The listing builds one solid part. Answer for the finished solid, in the listing's coordinates (mm). Face numbers are marked on the shaded views. A direction names the side the tool comes from. Coordinates: 2 decimals unless noted, no trailing zeros. Order: outer loops, then holes, each group sorted by start corner. A loop starts at its lowest first (then second) coordinate and runs counter-clockwise, first axis right, second up.
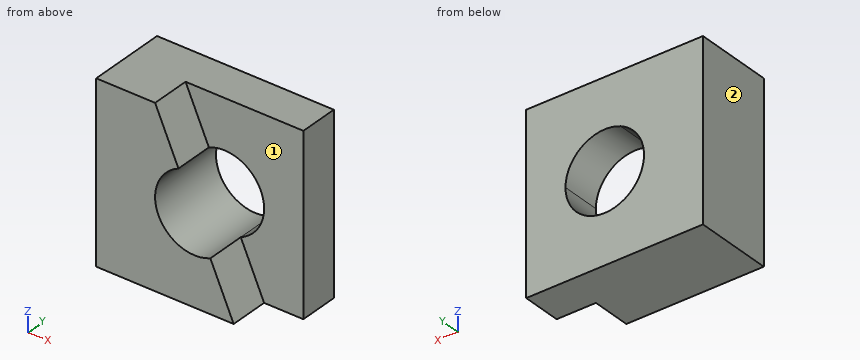
from build123d import *

# Parameters (mm, degrees)
F0_W     = 114.3
F0_H     = 114.3
F1_DEPTH = 25.4
F3_DEPTH = 25.4
F5_DEPTH = 50.801


with BuildPart() as f1:
    # F0 (on Front) → F1 (new body)
    with BuildSketch(Plane.XZ):
        with Locations((6.345086, -10.230491)):
            Rectangle(F0_W, F0_H)
    extrude(amount=F1_DEPTH)

    # F2 (on face) → F3 (join)
    with BuildSketch(Plane.XZ.offset(25.4)):
        Polygon((-12.704914, 46.919509), (-50.804914, 46.919509), (-50.804914, -67.380491), (38.095086, -67.380491), align=None)
    extrude(amount=F3_DEPTH)

    # F4 (on face) → F5 (cut, through all)
    with BuildSketch(Plane.XZ.offset(50.8)):
        with BuildLine():
            Line((23.011003, -33.441305), (2.379169, 12.980322))
            ThreePointArc((2.379169, 12.980322), (-10.515728, -20.546409), (23.011003, -33.441305))
        make_face()
        with BuildLine():
            ThreePointArc((23.011003, -33.441305), (33.992789, -24.071295), (38.095086, -10.230491))
            ThreePointArc((38.095086, -10.230491), (26.53589, 11.067211), (2.379169, 12.980322))
            Line((2.379169, 12.980322), (23.011003, -33.441305))
        make_face()
    extrude(amount=-F5_DEPTH, mode=Mode.SUBTRACT)


solid = f1.part
(1) Find section D-D on y = -38. Determine the outline of the cut face in (x, z).
(2) Find section C-C on z = -6.5. Determine the outline of the cut face in (x, y).
(3) A tool of negligible diameter and unlimited length cuts with its end or side. For the marked faces 1 and 2, from which of +Z, -Z, +X, -X, +Y, -Y can it reach the whole face along a straight path? Write none if from no direction.
(4) Find section A-A on y = -17.5. Determine the outline of the cut face in (x, z).
(5) Find section B-B on x = 29. Determine the outline of the cut face in (y, z).
(6) Find the intervals of material crossed by probe 1 along Y at (x, z) = (-4, 34); probe 2 along Z at (x, y) = (13.5, -11); probe 3 along X at (y, z) = (-18, -12), in increasing order.
(7) Given pin 1 Ø8 at (y, z) = (-39.5, -8) entering from +X; pin 2 Ø12 at (y, z) = (-38.5, -21) entering from +X, each flat-ended and moving along its own axis, determine where each tip first touches the part or whether it passes through.
Resolved:
1. outline: (-50.8, -67.38) - (38.1, -67.38) - (23.01, -33.44) arc R25.4 cw to (2.38, 12.98) - (-12.7, 46.92) - (-50.8, 46.92) - close
2. outline: (-50.8, -50.8) - (-12.43, -50.8) - (-12.43, 0) - (-50.8, 0) - close; (37.82, -25.4) - (63.5, -25.4) - (63.5, 0) - (37.82, 0) - close
3. face 1: +Z, +X, -Y
3. face 2: +Z, -Z, -X, +Y, -Y
4. outline: (-50.8, -67.38) - (63.5, -67.38) - (63.5, 46.92) - (-50.8, 46.92) - close; hole (23.01, -33.44) arc R25.4 ccw to (38.1, -10.23) arc R25.4 ccw (long way) to start
5. outline: (-50.8, -67.38) - (0, -67.38) - (0, -29.71) - (-25.4, -29.71) - (-25.4, -46.92) - (-50.8, -46.92) - close; (-25.4, 9.25) - (0, 9.25) - (0, 46.92) - (-25.4, 46.92) - close
6. probe 1: y = -25.4 to 0
6. probe 2: z = -67.38 to -35.62, 15.16 to 46.92
6. probe 3: x = -50.8 to -12.64, 38.03 to 63.5
7. pin 1: stops at x = -11.93
7. pin 2: stops at x = -6.38
